Autodesk Inventor part; units mm, degrees
ref_plane "YZ Plane" through (0, 0, 0) normal (1, 0, 0) x (0, 1, 0)
ref_plane "XZ Plane" through (0, 0, 0) normal (0, 1, 0) x (-1, 0, 0)
ref_plane "XY Plane" through (0, 0, 0) normal (0, 0, 1) x (1, 0, 0)
sketch "Sketch1" plane through (0, 0, 0) normal (0, 0, 1) x (1, 0, 0)
  circle A0 centre (0, 0) radius 14
  circle A1 centre (-4.25, 4.25) radius 1.1
  circle A2 centre (-4.25, -4.25) radius 1.1
  circle A3 centre (4.25, -4.25) radius 1.1
  circle A4 centre (4.25, 4.25) radius 1.1
  line L0 (-7.5, 11.8216) -> (-4, 40)
  line L1 (-4, 40) -> (4, 40)
  line L2 (4, 40) -> (7.5, 11.8216)
  point P0 (0, 40)
  dimension "d0" = 8.5
  dimension "d1" = 8.5
  dimension "d2" = 4.25
  dimension "d3" = 4.25
  dimension "d4" = 2.2
  dimension "d5" = 28
  dimension "d6" = 8
  dimension "d7" = 15
  dimension "d8" = 40
extrude "Extrusion1" add sketch "Sketch1" along normal blind 1
sketch "Sketch2" plane through (0, 0, 0) normal (0, 0, 1) x (1, 0, 0)
  line L0 (7.5, 11.8216) -> (4, 40)
  line L1 (4, 40) -> (-4, 40)
  line L2 (-4, 40) -> (-7.5, 11.8216)
  arc A0 (-7.5, 11.8216) -> (7.5, 11.8216) centre (0, 0) ccw
  circle A1 centre (-4.25, 4.25) radius 1.1
  circle A2 centre (-4.25, -4.25) radius 1.1
  circle A3 centre (4.25, -4.25) radius 1.1
  circle A4 centre (4.25, 4.25) radius 1.1
  circle A5 centre (-4.25, 4.25) radius 2
  circle A6 centre (-4.25, -4.25) radius 1.1
  circle A7 centre (-4.25, -4.25) radius 2
  circle A8 centre (4.25, -4.25) radius 1.1
  circle A9 centre (4.25, -4.25) radius 2
  circle A10 centre (4.25, 4.25) radius 2
  dimension "d11" = 4
extrude "Extrusion2" add sketch "Sketch2" against normal blind 2 contours A0 L2 L1 L0
chamfer "Chamfer1" distance 1.5 angle 45 2 edges at (-5.75, 25.9108, -2) (5.75, 25.9108, -2)
fillet "Fillet1" radius 1.5 1 edges at (0, -14, -2)
equation "\"d1\" = d0"
properties part number "Pointerlever"
Can you work these out from the model? Positions are in its coordinate system, mm. A direction names the side the tool comes from. Round coordinates to 2 decimals unless told otherwise and drop trailing zeros. Order: outer loops, then holes, each group sorted by start corner. A loop starts at its lowest first (then second) coordinate and runs counter-clockwise, first axis right, second up. Notation, with made-up numbers: (-27.5, 62.5) -> (9.5, 62.5) arc R17 ccw to (9.5, 95.5) -> close; hole circle Ø6 at (85.25, 84). An arc over 180 degrees is marked (long way). Return JSON: item names as keys, results as strings. Group by question number.
1. We'd pull the mould along X, two halves only. Please class faces 1 (the face through (0, 8, -2)), 2 (the face through (4, -6, 0)), 3 (the face through (-5.726, 26.108, 0.26)), 4 (the face through (-3, 3, 0)): released by +X, released by -X, zero draft, split by the parting line, or undercut.
2. I need wall thicknesses on line 1 (Y direction, x = 3.25, z = 0.15); line 2 (Y direction, x = 3.5, z = -0.35); line 3 (X direction, y = 5, z = 0.2). Which ranges of each line are inside material? Lowest first, please. Write a range as [from, to].
3. Which directions (+Z, -Z, +X, -X, +Y, -Y) give clear straight access to the entire face, cutting with the end or side of a thin tool? Please do faces 5 (the face through (5.774, 25.714, 0.26)), 6 (the face through (2.663, 3.033, -0.986)).
4. If we section it at A-A, the plane y = 14: Write out the boundary of the cut face in (x, z).
5. Will these pins go through, and if not, where does the flat tip stop? pin 1 (3 mm diameter, centred on x = 4.25, y = 4.25, fed in from -Z); pin 2 (1 mm diameter, centred on y = 2.5, z = -0.5, fed in from +X).
Output values:
{
 "1": {"face 1": "zero draft", "face 2": "undercut", "face 3": "released by -X", "face 4": "undercut"},
 "2": {"line 1": "[-13.62, -4.71], [-3.79, 3.79], [4.71, 40]", "line 2": "[-13.56, -6.1], [-2.4, 2.4], [6.1, 40]", "line 3": "[-13.08, -5.05], [-3.45, 3.45], [5.05, 13.08]"},
 "3": {"face 5": "+Z, -Z, +X, +Y", "face 6": "-Z"},
 "4": {"outline": "(-7.23, -0.5) -> (-5.72, -2) -> (5.72, -2) -> (7.23, -0.5) -> (7.23, 1) -> (-7.23, 1) -> close"},
 "5": {"pin 1": "z = 0", "pin 2": "x = 13.86"}
}
